```python
from build123d import *

# Parameters (mm, degrees)
IZIM1_R                     = 210
IZIM1_R_2                   = 200
Y_KSEKLIK_EKSTR_ZYON1_DEPTH = 10
KES_EKSTR_ZYON1_DEPTH       = 290
KES_EKSTR_ZYON1_DEPTH_BACK  = 290
KES_EKSTR_ZYON2_DEPTH       = 290
KES_EKSTR_ZYON2_DEPTH_BACK  = 290
KES_EKSTR_ZYON8_DEPTH       = 184
KES_EKSTR_ZYON8_DEPTH_BACK  = 455
IZIM6_W                     = 5
IZIM6_H                     = 10
Y_KSEKLIK_EKSTR_ZYON2_DEPTH = 10
IZIM7_W                     = 5
IZIM7_H                     = 10
Y_KSEKLIK_EKSTR_ZYON4_DEPTH = 10


with BuildPart() as part:
    # izim1 → Y_kseklik-Ekstr_zyon1 (new body)
    with BuildSketch(Plane.XY):
        Circle(IZIM1_R)
        Circle(IZIM1_R_2, mode=Mode.SUBTRACT)
    extrude(amount=Y_KSEKLIK_EKSTR_ZYON1_DEPTH)

    # izim3 → Kes-Ekstr_zyon1 (cut, two sides: drawn at the far end of the back side and taken through both)
    with BuildSketch(Plane(origin=(0, 0, 0), x_dir=(1, 0, 0), z_dir=(0, 1, 0)).offset(-KES_EKSTR_ZYON1_DEPTH_BACK)):
        with BuildLine():
            ThreePointArc((1, -5), (0.707106781, -4.292893219), (0, -4))
            Line((0, -4), (0, -6))
            ThreePointArc((0, -6), (0.707106781, -5.707106781), (1, -5))
        make_face()
        with BuildLine():
            Line((0, -6), (0, -4))
            ThreePointArc((0, -4), (-1, -5), (0, -6))
        make_face()
    extrude(amount=KES_EKSTR_ZYON1_DEPTH + KES_EKSTR_ZYON1_DEPTH_BACK, mode=Mode.SUBTRACT)

    # izim4 → Kes-Ekstr_zyon2 (cut, two sides: drawn at the far end of the back side and taken through both)
    with BuildSketch(Plane(origin=(0, 0, 0), x_dir=(0, 0, -1), z_dir=(1, 0, 0)).offset(-KES_EKSTR_ZYON2_DEPTH_BACK)):
        with BuildLine():
            ThreePointArc((-4, 0), (-5, 1), (-6, 0))
            Line((-6, 0), (-4, 0))
        make_face()
        with BuildLine():
            Line((-4, 0), (-6, 0))
            ThreePointArc((-6, 0), (-5, -1), (-4, 0))
        make_face()
    extrude(amount=KES_EKSTR_ZYON2_DEPTH + KES_EKSTR_ZYON2_DEPTH_BACK, mode=Mode.SUBTRACT)

    # izim5 → Kes-Ekstr_zyon8 (cut, two sides: drawn at the far end of the back side and taken through both)
    with BuildSketch(Plane.XY.offset(-KES_EKSTR_ZYON8_DEPTH_BACK)):
        with BuildLine():
            Line((-141.421356237, 141.421356237), (-148.492424049, 148.492424049))
            ThreePointArc((-148.492424049, 148.492424049), (0, -210), (148.492424049, 148.492424049))
            Line((148.492424049, 148.492424049), (141.421356237, 141.421356237))
            ThreePointArc((141.421356237, 141.421356237), (0, -200), (-141.421356237, 141.421356237))
        make_face()
    extrude(amount=KES_EKSTR_ZYON8_DEPTH + KES_EKSTR_ZYON8_DEPTH_BACK, mode=Mode.SUBTRACT)

    # izim6 → Y_kseklik-Ekstr_zyon2 (add)
    with BuildSketch(Plane(origin=(0, 0, 0), x_dir=(0, 0, -1), z_dir=(0.7071067811865477, -0.7071067811865475, 0))):
        with Locations((-2.5, 205)):
            Rectangle(IZIM6_W, IZIM6_H)
    extrude(amount=Y_KSEKLIK_EKSTR_ZYON2_DEPTH)

    # izim7 → Y_kseklik-Ekstr_zyon4 (add)
    with BuildSketch(Plane(origin=(0, 0, 0), x_dir=(0, 0, 1), z_dir=(-0.7071067811865477, -0.7071067811865475, 0))):
        with Locations((7.5, 205)):
            Rectangle(IZIM7_W, IZIM7_H)
    extrude(amount=Y_KSEKLIK_EKSTR_ZYON4_DEPTH)


solid = part.part
```
Model file for the job. Use its own axes, mm. A direction names the side the tool comes from. Coordinates: 2 decimals unless noted, no trailing zeros. Write each loop counter-clockwise with the first axis right and the second up, starting at its lowest first coordinate (ties: lowest second). Pieces come first, ordered by that corner, then holes. Notation, with made-up numbers: (-29.5, 82.25) - (20.5, 82.25) arc R23 ccw to (20.5, 104.25) - close; hole circle Ø7 at (6.5, 9). An arc over 180 degrees is marked (long way). One line per item, written item: value. Start each with the question number.
1. Slice it at C-C (x = 74). Write the cut outline in (y, z).
2. Probe line 1 (X direction, y = 177.5, z = 9.25); line 2 (X direction, y = 141.5, z = 1.5); line 3 (X direction, y = 141, z = 5.75). List the from-to ranges inside material, lowest first. Write a range as from..to.
3. Slice it at B-B (y = 159.5). Write the cut outline in (x, z).
4. Flat gauge pins, fed straight in: pin 1 (1.5 mm diameter, centred on y = 145.5, z = 3, fed in from +X); pin 2 (7 mm diameter, centred on x = 151, y = 142.5, fed in from +Z); pin 3 (4 mm diameter, centred on x = -66, z = 1, fed in from -Y). Where does each tip first touch, or does it go through?
5. Slice it at A-A (y = 194.5). Write the cut outline in (x, z).
6. Mould opens along X. For faces 4 (the flat face through (-144.907, 137.935, 7.465)), 5 (the flat face through (-152.08, 137.94, 7.46)), 6 (the flat face through (2, 201, 0)), 7 (the cylindrical face through (2.199, 199.988, 4.93)) say: released by +X, released by -X, zero draft, split by the parting line, or undercut.
7. Tool access for faces 1 (the flat face through (-148, 141, 5)), 2 (the flat face through (148, 141, 5)), 3 (the flat face through (144.907, 137.935, 2.535)): list every direction of +Z, -Z, +X, -X, +Y, -Y with a clear straight run to the whole face (end or side of a thin tool).
8. Slice it at D-D (x = 5). Write the cut outline in (y, z), plus the area to 3 significant figures.
Answers below:
1. outline: (185.81, 0) - (196.53, 0) - (196.53, 10) - (185.81, 10) - close
2. line 1: x = -112.22..-92.16, 92.16..112.22
2. line 2: x = -141.5..-141.34, 141.34..155.48
2. line 3: x = -155.14..-141.84
3. outline: (-136.6, 0) - (-120.66, 0) - (-120.66, 10) - (-136.6, 10) - close; (120.66, 0) - (136.6, 0) - (136.6, 10) - (120.66, 10) - close
4. pin 1: stops at x = 152.23
4. pin 2: stops at z = 5
4. pin 3: stops at y = 188.09
5. outline: (-79.18, 0) - (-46.58, 0) - (-46.58, 10) - (-79.18, 10) - close; (46.58, 0) - (79.18, 0) - (79.18, 10) - (46.58, 10) - close
6. face 4: released by +X
6. face 5: released by -X
6. face 6: zero draft
6. face 7: undercut
7. face 1: -Z, -X, -Y
7. face 2: +Z, +X, -Y
7. face 3: +Z, -Z, -X, -Y
8. outline: (199.94, 0) - (209.94, 0) - (209.94, 10) - (199.94, 10) - close
8. area: 100 mm^2
